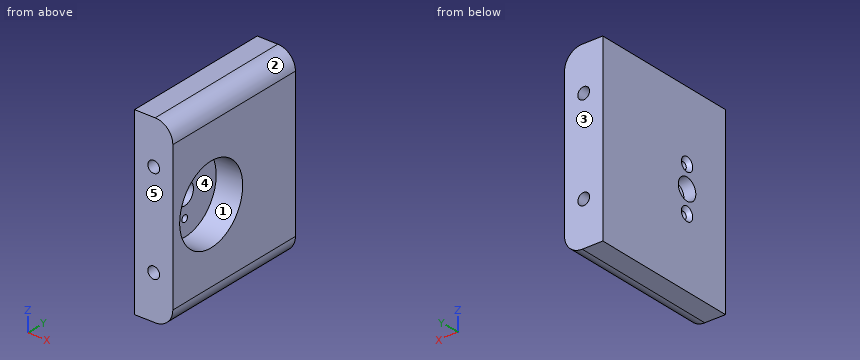
Autodesk Inventor part; units mm, degrees
ref_plane "YZ Plane" through (0, 0, 0) normal (1, 0, 0) x (0, 1, 0)
ref_plane "XZ Plane" through (0, 0, 0) normal (0, 1, 0) x (-1, 0, 0)
ref_plane "XY Plane" through (0, 0, 0) normal (0, 0, 1) x (1, 0, 0)
sketch "Эскиз1" plane through (0, 0, 0) normal (0, 1, 0) x (-1, 0, 0)
  line L0 (6.5, 31) -> (-6.5, 31)
  line L1 (-6.5, 31) -> (-6.5, -31)
  line L2 (-6.5, -31) -> (6.5, -31)
  line L3 (6.5, -31) -> (6.5, 31)
  line L4 (-6.5, 31) -> (6.5, -31) construction
  line L5 (0, 31) -> (0, -31) construction
  circle A0 centre (0, 16) radius 2
  line L6 (6.5, 0) -> (-6.5, 0) construction
  circle A1 centre (0, -16) radius 2
  point P0 (0, 0)
  point P1 (0, 0)
  dimension "d0" = 13
  dimension "d1" = 62
  dimension "d2" = 16
  dimension "d3" = 4
extrude "Выдавливание1" add sketch "Эскиз1" along normal blind 32
sketch "Эскиз2" plane through (6.5, 0, 31) normal (1, 0, 0) x (0, 0, -1)
  line L0 (0, 32) -> (62, 32)
  line L1 (62, 0) -> (0, 0)
  line L2 (62, 32) -> (0, 0) construction
  circle A0 centre (31, 16) radius 10.15
  line L3 (20.85, 16) -> (41.15, 16) construction
  circle A1 centre (23.5, 16) radius 1.15
  circle A2 centre (38.5, 16) radius 1.15
  line L4 (23.5, 16) -> (38.5, 16)
  circle A3 centre (31, 16) radius 13.15
  line L5 (31, 29.15) -> (31, 2.85)
  line L6 (62, 0) -> (62, 32)
  circle A4 centre (31, 16) radius 3.65
  point P0 (31, 0)
  dimension "d9" = 20.3
  dimension "d10" = 2.3
  dimension "d11" = 15
  dimension "d17" = 7.3
  dimension "d21" = 26.3
extrude "Выдавливание3" cut sketch "Эскиз2" against normal through all contours A2 | A1 | A4 L4 L5 | L5 L4 A4 | A4 L4 L5 | L5 L4 A4
extrude "Выдавливание4" cut sketch "Эскиз2" against normal blind 9
sketch "Эскиз3" plane through (0, 32, 0) normal (0, 1, 0) x (1, 0, 0)
  circle A0 centre (0, -16) radius 2
  circle A1 centre (0, 16) radius 2
  point P0 (0, 0)
extrude "Выдавливание5" add sketch "Эскиз3" against normal blind 25
fillet "Сопряжение1" radius 6 2 edges at (6.5, 16, 31) (6.5, 16, -31)
chamfer "Фаска1" distance 1.2 angle 45 2 edges at (-6.5, 16, -6.35) (-6.5, 16, 8.65)
sketch "Эскиз6" plane through (0, 32, 0) normal (0, 1, 0) x (1, 0, 0)
  arc A0 (6.5, 25) -> (0.5, 31) centre (0.5, 25) ccw
  line L0 (0.5, 31) -> (-6.5, 31)
  line L1 (-6.5, 31) -> (-6.5, -31)
  line L2 (-6.5, -31) -> (0.5, -31)
  arc A1 (0.5, -31) -> (6.5, -25) centre (0.5, -25) ccw
  line L3 (6.5, -25) -> (6.5, 25)
  point P0 (0, 0)
extrude "Выдавливание6" add sketch "Эскиз6" along normal blind 19.15
sketch "Эскиз7" plane through (0, 51.15, 0) normal (0, 1, 0) x (1, 0, 0)
  circle A0 centre (0, -16) radius 2
  circle A1 centre (0, 16) radius 2
  point P0 (0, 0)
extrude "Выдавливание7" cut sketch "Эскиз7" against normal blind 7
properties part number "motor_mount_edge" material "Полиэтилен, низкая плотность"
Input: part model. Units: mm. Frame: model coordinates. Face numbers are marked on the shaded views. A direction names the side the tool comes from. Round coordinates to 2 decimals unless told otherwise and drop trailing zeros. Loops run counter-clockwise (first coordinate to the right, second up) from the corner with the lowest first, then second, coordinate; pieces in that order, holes last. Notation, with made-up numbers: M 25.5,5.25 L 30.5,5.25 A23 cw 30.5,15.25 Z; hole C 33,-28 d11. An arc over 180 degrees is marked long. Answer in a Markdown table with one row per item. Add a question column.
1. Section D-D (z = 16). Output: boundary loops of the cut face in (x, y), and give its area (3 significant figures).
2. Contact query for flat-ended pins moving along their axis: pin 1 (2 mm diameter, centred on x = -0.5, z = -16, fed in from +Y); pin 2 (1.2 mm diameter, centred on x = 0.5, z = -15.5, fed in from -Y); pin 3 (3.5 mm diameter, centred on y = 16, z = -7.5, fed in from -X); pin 4 (2 mm diameter, centred on y = 16, z = 7.5, fed in from -X). Output: stop coordinate, or through.
3. Ray query, probe 1 along Z at (x, y) = (0, 46); probe 2 along X at (y, z) = (48.75, 16); probe 3 along Y at (x, z) = (-5.3, 0). Return the intervals inside material, ascending.
4. Section B-B (z = 0). Output: boundary loops of the cut face in (x, y).
5. Section C-C (y = 45.5). Output: boundary loops of the cut face in (x, z).
6. Section A-A (y = 16). Output: boundary loops of the cut face in (x, z), and give its area (3 significant figures).
7. Set-up query: the marked faces 4 and 5. Return all of +Z, -Z, +X, -X, +Y, -Y with unobstructed straight access to the full face (end or side cutting, diameter ignored); none if empty.
8. Mould query, pull axis Y, two halves, no side actions, for the marked faces 1, 2 and 3. Classes: released by +Y, released by -Y, zero draft, split by the parting line, or undercut.
Values follow:
| question | item | result |
|---|---|---|
| 1 | outline | M -6.5,0 L -2,0 L -2,7 L 2,7 L 2,0 L 6.5,0 L 6.5,51.15 L 2,51.15 L 2,44.15 L -2,44.15 L -2,51.15 L -6.5,51.15 Z |
| 1 | area | 609 mm^2 |
| 2 | pin 1 | y = 44.15 |
| 2 | pin 2 | y = 7 |
| 2 | pin 3 | x = -5.9 |
| 2 | pin 4 | through |
| 3 | probe 1 | -31 to -18, -14 to 14, 18 to 31 |
| 3 | probe 2 | -6.5 to -2, 2 to 6.5 |
| 3 | probe 3 | 0 to 12.35, 19.65 to 51.15 |
| 4 | outline | M -6.5,0 L 6.5,0 L 6.5,2.85 L -2.5,2.85 L -2.5,12.35 L -6.5,12.35 Z; M -6.5,19.65 L -2.5,19.65 L -2.5,29.15 L 6.5,29.15 L 6.5,51.15 L -6.5,51.15 Z |
| 5 | outline | M -6.5,-31 L 0.5,-31 A6 ccw 6.5,-25 L 6.5,25 A6 ccw 0.5,31 L -6.5,31 Z; hole C 0,-16 d4; hole C 0,16 d4 |
| 6 | outline | M -6.5,-31 L 0.5,-31 A6 ccw 6.5,-25 L 6.5,-13.15 L -2.5,-13.15 L -2.5,-8.65 L -5.3,-8.65 L -6.5,-9.85 Z; M -6.5,-5.15 L -5.3,-6.35 L -2.5,-6.35 L -2.5,-3.65 L -6.5,-3.65 Z; M -6.5,3.65 L -2.5,3.65 L -2.5,6.35 L -5.3,6.35 L -6.5,5.15 Z; M -6.5,9.85 L -5.3,8.65 L -2.5,8.65 L -2.5,13.15 L 6.5,13.15 L 6.5,25 A6 ccw 0.5,31 L -6.5,31 Z |
| 6 | area | 503 mm^2 |
| 7 | face 4 | +X |
| 7 | face 5 | +Z, -Z, +X, -X, -Y |
| 8 | face 1 | undercut |
| 8 | face 2 | zero draft |
| 8 | face 3 | released by +Y |
